Part model, mm, in its own coordinate system. A direction names the side the tool comes from. Give positions to 0.01 mm unless a question says otherwise; leave off trailing zeros. Order: outer loops, then holes, each group sorted by start corner. A loop starts at its lowest first (then second) coordinate and runs counter-clockwise, first axis right, second up. Notation, with made-up numbers: M 1,43 L 6,43 A10 cw 6,51 Z; hole C 54.5,-10 d10. An arc over 180 degrees is marked long. Answer as a JSON object with one key per item and string values.
from build123d import *

# Parameters (mm, degrees)
SKETCH_1_R            = 1.55
EXTRUDE_514_DEPTH     = 2.5
EXTRUDE_START         = 2.5
EXTRUDE_981_DEPTH     = 7.5
SKETCH_3_W            = 4.5
SKETCH_3_H            = 12.978713764
EXTRUDE_1_DEPTH       = 9.75
CHAMFER_1_SIZE        = 1
FILLET_5_R            = 0.75
CUT_EXTRUDE_1_DEPTH   = 2
SKETCH_7_R            = 1.55
CUT_EXTRUDE_2_DEPTH   = 4.5
EXTRUDE_2642_DEPTH    = 7.25
CUT_EXTRUDE_1_2_DEPTH = 26.037686694
EXTRUDE_START_2       = 1.5
SKETCH_9_R            = 1.55
EXTRUDE_2_DEPTH       = 1.5
FILLET_6_R            = 0.25


with BuildPart() as part:
    # 草图1 → Extrude 514 (new body)
    with BuildSketch(Plane(origin=(0, 0, 0), x_dir=(1, 0, 0), z_dir=(0, 1, 0))):
        with BuildLine():
            Line((-10.1243866, 13.845154317), (6.15423406, 2.01804411))
            ThreePointArc((6.15423406, 2.01804411), (7.315700706, -5.315167685), (-0.017511089, -6.476634331))
            Line((-0.017511089, -6.476634331), (-10.1243866, 0.866440553))
            Line((-10.1243866, 0.866440553), (-10.1243866, 13.845154317))
        make_face()
        with Locations(Location((0, 0, 0), (0, 0, 270))):
            Circle(SKETCH_1_R, mode=Mode.SUBTRACT)
    extrude(amount=EXTRUDE_514_DEPTH)

    # 草图2 → Extrude 981 (add)
    with BuildSketch(Plane(origin=(0, 0, 0), x_dir=(1, 0, 0), z_dir=(0, 1, 0)).offset(EXTRUDE_START)):
        Polygon((-10.1243866, 0.866440553), (-0.017511089, -6.476634331), (-1.193081594, -8.09466832), (-11.299957105, -0.751593436), align=None)
        Polygon((7.329804565, 3.636078099), (-0.809505765, 9.549633202), (-1.98507627, 7.931599213), (6.15423406, 2.01804411), align=None)
    extrude(amount=-EXTRUDE_981_DEPTH)

    # 草图3 → 限位-1 (add)
    with BuildSketch(Plane(origin=(0, 0, 0), x_dir=(1, 0, 0), z_dir=(0, 1, 0))):
        with Locations((-12.3743866, 7.355797435)):
            Rectangle(SKETCH_3_W, SKETCH_3_H)
    extrude(amount=EXTRUDE_1_DEPTH)

    # 倒角1
    chamfer_1_edges = [part.edges().sort_by_distance(p)[0] for p in [
        (0, 0, -1.55),
        (0, 2.5, -1.55),
    ]]
    chamfer(chamfer_1_edges, length=CHAMFER_1_SIZE)

    # 圆角5
    fillet_5_edges = [part.edges().sort_by_distance(p)[0] for p in [
        (-1.193081594, -1.25, 8.09466832),
        (-11.299957105, -1.25, 0.751593436),
        (-1.98507627, 1.25, -7.931599213),
        (-0.809505765, -1.25, -9.549633202),
        (7.329804565, -1.25, -3.636078099),
        (-0.017511089, 1.25, 6.476634331),
        (6.15423406, 1.25, -2.01804411),
    ]]
    fillet(fillet_5_edges, radius=FILLET_5_R)

    # 草图5 → Cut-Extrude 1 (cut)
    with BuildSketch(Plane(origin=(-10.1243866, 0, 0), x_dir=(0, 0, -1), z_dir=(1, 0, 0))):
        Polygon((10.560091429, 5.75), (8.957944432, 8.525), (5.753650438, 8.525), (4.151503441, 5.75), (5.753650438, 2.975), (8.957944432, 2.975), align=None)
    extrude(amount=-CUT_EXTRUDE_1_DEPTH, mode=Mode.SUBTRACT)

    # 草图7 → 切除-拉伸2 (cut)
    with BuildSketch(Plane(origin=(-10.1243866, 0, 0), x_dir=(0, 0, -1), z_dir=(1, 0, 0))):
        with Locations((7.355797435, 5.75)):
            Circle(SKETCH_7_R)
    extrude(amount=-CUT_EXTRUDE_2_DEPTH, mode=Mode.SUBTRACT)

    # 草图8 → Extrude 2642 (add)
    with BuildSketch(Plane(origin=(0, 0, 0), x_dir=(1, 0, 0), z_dir=(0, 1, 0)).offset(EXTRUDE_START)):
        Polygon((-10.1243866, 13.845154317), (-8.6243866, 12.755340525), (-8.6243866, 0.866440553), (-10.1243866, 0.866440553), align=None)
    extrude(amount=EXTRUDE_2642_DEPTH)

    # 草图5<2> → Cut-Extrude 1 2 (cut, through all)
    with BuildSketch(Plane(origin=(-10.1243866, 0, 0), x_dir=(0, 0, -1), z_dir=(1, 0, 0))):
        Polygon((10.560091429, 5.75), (8.957944432, 8.525), (5.753650438, 8.525), (4.151503441, 5.75), (5.753650438, 2.975), (8.957944432, 2.975), align=None)
    extrude(amount=CUT_EXTRUDE_1_2_DEPTH, mode=Mode.SUBTRACT)

    # 草图9 → 结构补强螺母位-2 (add)
    with BuildSketch(Plane(origin=(-12.1243866, 0, 0), x_dir=(0, 0, -1), z_dir=(1, 0, 0)).offset(EXTRUDE_START_2)):
        Polygon((8.957944432, 2.975), (10.560091429, 5.75), (8.957944432, 8.525), (5.753650438, 8.525), (4.151503441, 5.75), (5.753650438, 2.975), align=None)
        with Locations((7.355797435, 5.75)):
            Circle(SKETCH_9_R, mode=Mode.SUBTRACT)
    extrude(amount=-EXTRUDE_2_DEPTH)

    # 圆角6
    fillet_6_edges = [part.edges().sort_by_distance(p)[0] for p in [
        (-10.1243866, 1.25, -0.866440553),
    ]]
    fillet(fillet_6_edges, radius=FILLET_6_R)


solid = part.part
1. Which spindle directions (+Z, -Z, +X, -X, +Y, -Y) get a long thin tool onto all of the face, cutting with end or side? Do faces 5 (the flat face through (6.52, -2.03, -2.52)), 6 (the flat face through (-8.624, 6, -4)), 7 (the flat face through (-9.638, 4.343, -9.748)). Say none if no direction does.
Worked answers:
{"face 5": "+X, -Y", "face 6": "+Z, -Z, +X, +Y", "face 7": "+X"}
2. Cut at B-B on x = -12.25. Give the cut face in (y, z), plus the area to 3 significant figures.
Worked answers:
{"outline": "M 0,-13.85 L 9.75,-13.85 L 9.75,-0.87 L 0,-0.87 Z; hole C 5.75,-7.36 d3.1", "area": "119 mm^2"}
3. Pin check, flat tips, straight feed: P1, Ø2, axis at x = -9.5, z = -7.5, coming from the -Y side; P2, Ø2, axis at y = 6, z = -6.5, coming from the +X side; P3, Ø1, axis at x = 0.5, y = 2, coming from the -Z side. Stop position of each tip, or through.
Worked answers:
{"P1": "stops at y = 0", "P2": "stops at x = -10.62", "P3": "stops at z = -8.96"}
4. Probe line 1 along Y through (x, z) = (-0.5, -6.5); line 2 along X through (y, z) = (8.25, -5.75); line 3 along X through (y, z) = (2.75, -1). List the from-to ranges inside material, lowest first.
Worked answers:
{"line 1": "y = 0 to 2.5", "line 2": "x = -14.62 to -10.62", "line 3": "x = -14.62 to -8.62"}
5. Cut at D-D on y = 7.75. Give the cut face in (x, z), plus the area to 3 significant figures.
Worked answers:
{"outline": "M -14.62,-13.85 L -10.12,-13.85 L -8.62,-12.76 L -8.62,-9.41 L -10.62,-9.41 L -10.62,-5.31 L -8.62,-5.31 L -8.62,-0.87 L -14.62,-0.87 Z", "area": "68.9 mm^2"}
6. Two-plate mould, pull along Z, no slides. Class faces 1 (the flat face through (3, -5, -6)), 2 (the flat face through (3.309, -1.197, -6.558)), 3 (the flat face through (-10, 2.975, -7)), 4 (the flat face through (-10, 8.525, -7)): +Z half, -Z half, draft (parallel to the pull), parting line (faces both ways), or undercut.
Worked answers:
{"face 1": "draft", "face 2": "-Z half", "face 3": "undercut", "face 4": "undercut"}
7. Cut at A-A on y = -1. Give the cut face in (x, z).
Worked answers:
{"outline": "M -10.86,0.14 L -10.12,-0.87 L -0.02,6.48 L -0.75,7.49 A0.75 ccw -1.8,7.65 L -10.69,1.19 A0.75 ccw Z; M -1.99,-7.93 L -1.25,-8.94 A0.75 ccw -0.2,-9.11 L 6.72,-4.08 A0.75 ccw 6.89,-3.03 L 6.15,-2.02 Z"}
8. Cut at C-C on z = -7.25. Give the cut face in (x, y) (3 decimals).
Worked answers:
{"outline": "M -14.624,0 L -1.047,0 L -1.047,-5 L 2.356,-5 L 2.356,2.5 L -8.624,2.5 L -8.624,2.975 L -10.624,2.975 L -10.624,4.204 L -14.624,4.204 Z; M -14.624,7.296 L -10.624,7.296 L -10.624,8.525 L -8.624,8.525 L -8.624,9.75 L -14.624,9.75 Z"}
